Read the model definition and answer for the solid it produces. Units are mm, in the model's axes. A direction names the side the tool comes from. Coordinates: 2 decimals unless noted, no trailing zeros. Write each loop counter-clockwise with the first axis right and the second up, starting at its lowest first coordinate (ties: lowest second). Pieces come first, ordered by that corner, then holes. Notation, with made-up numbers: (40, -12.5) -> (79, -12.5) arc R13 cw to (79, -0.5) -> close; hole circle Ø10 at (-40, 56). An arc over 180 degrees is marked (long way). Answer in a Markdown table with one row per item. Add a question column.
Item 1: Which of the six approach directions +Z, -Z, +X, -X, +Y, -Y give full straight-line access (tool end or side, diameter ignored) to faces 1 (the face through (122, 13, -12.446)), 2 (the face through (122, 13, 10.414))?
Item 2: Section B-B on x = 267 is taken. Write down the section's boundary in (y, z), then the cut area to 3 significant figures.
Item 3: Given pin 1 Ø4 at (x, y) = (281.178, 12.7) entering from +Z, flat-ended and moving along its own axis, determine where the tip first touches the part or whether it passes through.
Item 4: For a pull along Y with two mould halves and no side action, classify faces 3 (the face through (122, 13, 12.954)), 4 (the face through (-75.18, 8.26, -11.16)), 5 (the face through (122, 2.54, 0)), 6 (the face through (122, 0, 0)) as +Y half, -Y half, draft (parallel to the pull), parting line (faces both ways), or undercut.
Item 5: Straight lines are drawn through the part: line 1 (Y direction, x = 123, z = -2.75); line 2 (Z direction, x = 214, y = 8.25); line 3 (X direction, y = 9, z = -11). For each, find the intervals that lie inside material, in ascending order. Write a range as from..to.
Item 6: Section A-A on z = -5.5 is taken. Write down the section's boundary in (x, y), then the cut area to 3 significant figures.
```python
from build123d import *

# Parameters (mm, degrees)
SKETCH1_W           = 431.8
SKETCH1_H           = 25.4
BOSS_EXTRUDE1_DEPTH = 25.4
SKETCH2_W           = 20.32
SKETCH2_H           = 20.32
CUT_EXTRUDE1_DEPTH  = 433.740344914
CUT_EXTRUDE2_REACH  = 344.058
SKETCH3_R           = 1.5875
CUT_EXTRUDE3_REACH  = 344.755
SKETCH4_R           = 3.175
SKETCH4_R_2         = 3.302


with BuildPart() as part:
    # Sketch1 → Boss-Extrude1 (new body)
    with BuildSketch(Plane(origin=(0, 0, 0), x_dir=(1, 0, 0), z_dir=(0, 1, 0))):
        with Locations((124.968, -0.254)):
            Rectangle(SKETCH1_W, SKETCH1_H)
    extrude(amount=BOSS_EXTRUDE1_DEPTH)

    # Sketch2 → Cut-Extrude1 (cut, through all)
    with BuildSketch(Plane.ZY.offset(90.932)):
        with Locations((0.254, 12.7)):
            Rectangle(SKETCH2_W, SKETCH2_H)
    extrude(amount=-CUT_EXTRUDE1_DEPTH, mode=Mode.SUBTRACT)

    # Cut-Extrude2: up to this face of the body (flat: up to its plane)
    cut_extrude2_end = Plane(part.part.faces().sort_by_distance((124.968, 12.7, -12.446))[0])
    # Sketch3 → Cut-Extrude2 (cut, up to the picked face)
    with BuildSketch(Plane(origin=(0, 12.446, 12.954), x_dir=(1, 0, 0), z_dir=(0, 0, -1)), mode=Mode.PRIVATE) as cut_extrude2_sk1:
        with Locations((-74.422, -0.254)):
            Circle(SKETCH3_R)
    cut_extrude2_tool1 = split(extrude(cut_extrude2_sk1.sketch, amount=CUT_EXTRUDE2_REACH, mode=Mode.PRIVATE), bisect_by=cut_extrude2_end, keep=Keep.BOTH, mode=Mode.PRIVATE)
    # Sketch3 → Cut-Extrude2 (cut, up to the picked face)
    with BuildSketch(Plane(origin=(0, 12.446, 12.954), x_dir=(1, 0, 0), z_dir=(0, 0, -1)), mode=Mode.PRIVATE) as cut_extrude2_sk2:
        with Locations((-49.022, -0.254)):
            Circle(SKETCH3_R)
    cut_extrude2_tool2 = split(extrude(cut_extrude2_sk2.sketch, amount=CUT_EXTRUDE2_REACH, mode=Mode.PRIVATE), bisect_by=cut_extrude2_end, keep=Keep.BOTH, mode=Mode.PRIVATE)
    # Sketch3 → Cut-Extrude2 (cut, up to the picked face)
    with BuildSketch(Plane(origin=(0, 12.446, 12.954), x_dir=(1, 0, 0), z_dir=(0, 0, -1)), mode=Mode.PRIVATE) as cut_extrude2_sk3:
        with Locations((-23.622, -0.254)):
            Circle(SKETCH3_R)
    cut_extrude2_tool3 = split(extrude(cut_extrude2_sk3.sketch, amount=CUT_EXTRUDE2_REACH, mode=Mode.PRIVATE), bisect_by=cut_extrude2_end, keep=Keep.BOTH, mode=Mode.PRIVATE)
    # Sketch3 → Cut-Extrude2 (cut, up to the picked face)
    with BuildSketch(Plane(origin=(0, 12.446, 12.954), x_dir=(1, 0, 0), z_dir=(0, 0, -1)), mode=Mode.PRIVATE) as cut_extrude2_sk4:
        with Locations((1.778, -0.254)):
            Circle(SKETCH3_R)
    cut_extrude2_tool4 = split(extrude(cut_extrude2_sk4.sketch, amount=CUT_EXTRUDE2_REACH, mode=Mode.PRIVATE), bisect_by=cut_extrude2_end, keep=Keep.BOTH, mode=Mode.PRIVATE)
    # Sketch3 → Cut-Extrude2 (cut, up to the picked face)
    with BuildSketch(Plane(origin=(0, 12.446, 12.954), x_dir=(1, 0, 0), z_dir=(0, 0, -1)), mode=Mode.PRIVATE) as cut_extrude2_sk5:
        with Locations((27.178, -0.254)):
            Circle(SKETCH3_R)
    cut_extrude2_tool5 = split(extrude(cut_extrude2_sk5.sketch, amount=CUT_EXTRUDE2_REACH, mode=Mode.PRIVATE), bisect_by=cut_extrude2_end, keep=Keep.BOTH, mode=Mode.PRIVATE)
    # Sketch3 → Cut-Extrude2 (cut, up to the picked face)
    with BuildSketch(Plane(origin=(0, 12.446, 12.954), x_dir=(1, 0, 0), z_dir=(0, 0, -1)), mode=Mode.PRIVATE) as cut_extrude2_sk6:
        with Locations((52.578, -0.254)):
            Circle(SKETCH3_R)
    cut_extrude2_tool6 = split(extrude(cut_extrude2_sk6.sketch, amount=CUT_EXTRUDE2_REACH, mode=Mode.PRIVATE), bisect_by=cut_extrude2_end, keep=Keep.BOTH, mode=Mode.PRIVATE)
    # Sketch3 → Cut-Extrude2 (cut, up to the picked face)
    with BuildSketch(Plane(origin=(0, 12.446, 12.954), x_dir=(1, 0, 0), z_dir=(0, 0, -1)), mode=Mode.PRIVATE) as cut_extrude2_sk7:
        with Locations((77.978, -0.254)):
            Circle(SKETCH3_R)
    cut_extrude2_tool7 = split(extrude(cut_extrude2_sk7.sketch, amount=CUT_EXTRUDE2_REACH, mode=Mode.PRIVATE), bisect_by=cut_extrude2_end, keep=Keep.BOTH, mode=Mode.PRIVATE)
    # Sketch3 → Cut-Extrude2 (cut, up to the picked face)
    with BuildSketch(Plane(origin=(0, 12.446, 12.954), x_dir=(1, 0, 0), z_dir=(0, 0, -1)), mode=Mode.PRIVATE) as cut_extrude2_sk8:
        with Locations((103.378, -0.254)):
            Circle(SKETCH3_R)
    cut_extrude2_tool8 = split(extrude(cut_extrude2_sk8.sketch, amount=CUT_EXTRUDE2_REACH, mode=Mode.PRIVATE), bisect_by=cut_extrude2_end, keep=Keep.BOTH, mode=Mode.PRIVATE)
    # Sketch3 → Cut-Extrude2 (cut, up to the picked face)
    with BuildSketch(Plane(origin=(0, 12.446, 12.954), x_dir=(1, 0, 0), z_dir=(0, 0, -1)), mode=Mode.PRIVATE) as cut_extrude2_sk9:
        with Locations((128.778, -0.254)):
            Circle(SKETCH3_R)
    cut_extrude2_tool9 = split(extrude(cut_extrude2_sk9.sketch, amount=CUT_EXTRUDE2_REACH, mode=Mode.PRIVATE), bisect_by=cut_extrude2_end, keep=Keep.BOTH, mode=Mode.PRIVATE)
    # Sketch3 → Cut-Extrude2 (cut, up to the picked face)
    with BuildSketch(Plane(origin=(0, 12.446, 12.954), x_dir=(1, 0, 0), z_dir=(0, 0, -1)), mode=Mode.PRIVATE) as cut_extrude2_sk10:
        with Locations((154.178, -0.254)):
            Circle(SKETCH3_R)
    cut_extrude2_tool10 = split(extrude(cut_extrude2_sk10.sketch, amount=CUT_EXTRUDE2_REACH, mode=Mode.PRIVATE), bisect_by=cut_extrude2_end, keep=Keep.BOTH, mode=Mode.PRIVATE)
    # Sketch3 → Cut-Extrude2 (cut, up to the picked face)
    with BuildSketch(Plane(origin=(0, 12.446, 12.954), x_dir=(1, 0, 0), z_dir=(0, 0, -1)), mode=Mode.PRIVATE) as cut_extrude2_sk11:
        with Locations((179.578, -0.254)):
            Circle(SKETCH3_R)
    cut_extrude2_tool11 = split(extrude(cut_extrude2_sk11.sketch, amount=CUT_EXTRUDE2_REACH, mode=Mode.PRIVATE), bisect_by=cut_extrude2_end, keep=Keep.BOTH, mode=Mode.PRIVATE)
    # Sketch3 → Cut-Extrude2 (cut, up to the picked face)
    with BuildSketch(Plane(origin=(0, 12.446, 12.954), x_dir=(1, 0, 0), z_dir=(0, 0, -1)), mode=Mode.PRIVATE) as cut_extrude2_sk12:
        with Locations((204.978, -0.254)):
            Circle(SKETCH3_R)
    cut_extrude2_tool12 = split(extrude(cut_extrude2_sk12.sketch, amount=CUT_EXTRUDE2_REACH, mode=Mode.PRIVATE), bisect_by=cut_extrude2_end, keep=Keep.BOTH, mode=Mode.PRIVATE)
    # Sketch3 → Cut-Extrude2 (cut, up to the picked face)
    with BuildSketch(Plane(origin=(0, 12.446, 12.954), x_dir=(1, 0, 0), z_dir=(0, 0, -1)), mode=Mode.PRIVATE) as cut_extrude2_sk13:
        with Locations((230.378, -0.254)):
            Circle(SKETCH3_R)
    cut_extrude2_tool13 = split(extrude(cut_extrude2_sk13.sketch, amount=CUT_EXTRUDE2_REACH, mode=Mode.PRIVATE), bisect_by=cut_extrude2_end, keep=Keep.BOTH, mode=Mode.PRIVATE)
    # Sketch3 → Cut-Extrude2 (cut, up to the picked face)
    with BuildSketch(Plane(origin=(0, 12.446, 12.954), x_dir=(1, 0, 0), z_dir=(0, 0, -1)), mode=Mode.PRIVATE) as cut_extrude2_sk14:
        with Locations((255.778, -0.254)):
            Circle(SKETCH3_R)
    cut_extrude2_tool14 = split(extrude(cut_extrude2_sk14.sketch, amount=CUT_EXTRUDE2_REACH, mode=Mode.PRIVATE), bisect_by=cut_extrude2_end, keep=Keep.BOTH, mode=Mode.PRIVATE)
    # Sketch3 → Cut-Extrude2 (cut, up to the picked face)
    with BuildSketch(Plane(origin=(0, 12.446, 12.954), x_dir=(1, 0, 0), z_dir=(0, 0, -1)), mode=Mode.PRIVATE) as cut_extrude2_sk15:
        with Locations((281.178, -0.254)):
            Circle(SKETCH3_R)
    cut_extrude2_tool15 = split(extrude(cut_extrude2_sk15.sketch, amount=CUT_EXTRUDE2_REACH, mode=Mode.PRIVATE), bisect_by=cut_extrude2_end, keep=Keep.BOTH, mode=Mode.PRIVATE)
    # Sketch3 → Cut-Extrude2 (cut, up to the picked face)
    with BuildSketch(Plane(origin=(0, 12.446, 12.954), x_dir=(1, 0, 0), z_dir=(0, 0, -1)), mode=Mode.PRIVATE) as cut_extrude2_sk16:
        with Locations((306.578, -0.254)):
            Circle(SKETCH3_R)
    cut_extrude2_tool16 = split(extrude(cut_extrude2_sk16.sketch, amount=CUT_EXTRUDE2_REACH, mode=Mode.PRIVATE), bisect_by=cut_extrude2_end, keep=Keep.BOTH, mode=Mode.PRIVATE)
    # Sketch3 → Cut-Extrude2 (cut, up to the picked face)
    with BuildSketch(Plane(origin=(0, 12.446, 12.954), x_dir=(1, 0, 0), z_dir=(0, 0, -1)), mode=Mode.PRIVATE) as cut_extrude2_sk17:
        with Locations((331.978, -0.254)):
            Circle(SKETCH3_R)
    cut_extrude2_tool17 = split(extrude(cut_extrude2_sk17.sketch, amount=CUT_EXTRUDE2_REACH, mode=Mode.PRIVATE), bisect_by=cut_extrude2_end, keep=Keep.BOTH, mode=Mode.PRIVATE)
    add(cut_extrude2_tool1.solids().sort_by(Axis((-74.422, 12.7, 12.954), (0, 0, -1)))[0], mode=Mode.SUBTRACT)
    add(cut_extrude2_tool2.solids().sort_by(Axis((-49.022, 12.7, 12.954), (0, 0, -1)))[0], mode=Mode.SUBTRACT)
    add(cut_extrude2_tool3.solids().sort_by(Axis((-23.622, 12.7, 12.954), (0, 0, -1)))[0], mode=Mode.SUBTRACT)
    add(cut_extrude2_tool4.solids().sort_by(Axis((1.778, 12.7, 12.954), (0, 0, -1)))[0], mode=Mode.SUBTRACT)
    add(cut_extrude2_tool5.solids().sort_by(Axis((27.178, 12.7, 12.954), (0, 0, -1)))[0], mode=Mode.SUBTRACT)
    add(cut_extrude2_tool6.solids().sort_by(Axis((52.578, 12.7, 12.954), (0, 0, -1)))[0], mode=Mode.SUBTRACT)
    add(cut_extrude2_tool7.solids().sort_by(Axis((77.978, 12.7, 12.954), (0, 0, -1)))[0], mode=Mode.SUBTRACT)
    add(cut_extrude2_tool8.solids().sort_by(Axis((103.378, 12.7, 12.954), (0, 0, -1)))[0], mode=Mode.SUBTRACT)
    add(cut_extrude2_tool9.solids().sort_by(Axis((128.778, 12.7, 12.954), (0, 0, -1)))[0], mode=Mode.SUBTRACT)
    add(cut_extrude2_tool10.solids().sort_by(Axis((154.178, 12.7, 12.954), (0, 0, -1)))[0], mode=Mode.SUBTRACT)
    add(cut_extrude2_tool11.solids().sort_by(Axis((179.578, 12.7, 12.954), (0, 0, -1)))[0], mode=Mode.SUBTRACT)
    add(cut_extrude2_tool12.solids().sort_by(Axis((204.978, 12.7, 12.954), (0, 0, -1)))[0], mode=Mode.SUBTRACT)
    add(cut_extrude2_tool13.solids().sort_by(Axis((230.378, 12.7, 12.954), (0, 0, -1)))[0], mode=Mode.SUBTRACT)
    add(cut_extrude2_tool14.solids().sort_by(Axis((255.778, 12.7, 12.954), (0, 0, -1)))[0], mode=Mode.SUBTRACT)
    add(cut_extrude2_tool15.solids().sort_by(Axis((281.178, 12.7, 12.954), (0, 0, -1)))[0], mode=Mode.SUBTRACT)
    add(cut_extrude2_tool16.solids().sort_by(Axis((306.578, 12.7, 12.954), (0, 0, -1)))[0], mode=Mode.SUBTRACT)
    add(cut_extrude2_tool17.solids().sort_by(Axis((331.978, 12.7, 12.954), (0, 0, -1)))[0], mode=Mode.SUBTRACT)

    # Cut-Extrude3: up to this face of the body (flat: up to its plane)
    cut_extrude3_end = Plane(part.part.faces().sort_by_distance((124.920663358, 12.7, -12.446))[0])
    # Sketch4 → Cut-Extrude3 (cut, up to the picked face)
    with BuildSketch(Plane.XY.offset(12.954), mode=Mode.PRIVATE) as cut_extrude3_sk1:
        with Locations((329.438, 12.763758165)):
            Circle(SKETCH4_R)
    cut_extrude3_tool1 = split(extrude(cut_extrude3_sk1.sketch, amount=-CUT_EXTRUDE3_REACH, mode=Mode.PRIVATE), bisect_by=cut_extrude3_end, keep=Keep.BOTH, mode=Mode.PRIVATE)
    # Sketch4 → Cut-Extrude3 (cut, up to the picked face)
    with BuildSketch(Plane.XY.offset(12.954), mode=Mode.PRIVATE) as cut_extrude3_sk2:
        with Locations((-78.232, 9.525)):
            Circle(SKETCH4_R_2)
    cut_extrude3_tool2 = split(extrude(cut_extrude3_sk2.sketch, amount=-CUT_EXTRUDE3_REACH, mode=Mode.PRIVATE), bisect_by=cut_extrude3_end, keep=Keep.BOTH, mode=Mode.PRIVATE)
    # Sketch4 → Cut-Extrude3 (cut, up to the picked face)
    with BuildSketch(Plane.XY.offset(12.954), mode=Mode.PRIVATE) as cut_extrude3_sk3:
        with Locations((-52.832, 9.525)):
            Circle(SKETCH4_R_2)
    cut_extrude3_tool3 = split(extrude(cut_extrude3_sk3.sketch, amount=-CUT_EXTRUDE3_REACH, mode=Mode.PRIVATE), bisect_by=cut_extrude3_end, keep=Keep.BOTH, mode=Mode.PRIVATE)
    add(cut_extrude3_tool1.solids().sort_by(Axis((329.438, 12.763758, 12.954), (0, 0, -1)))[0], mode=Mode.SUBTRACT)
    add(cut_extrude3_tool2.solids().sort_by(Axis((-78.232, 9.525, 12.954), (0, 0, -1)))[0], mode=Mode.SUBTRACT)
    add(cut_extrude3_tool3.solids().sort_by(Axis((-52.832, 9.525, 12.954), (0, 0, -1)))[0], mode=Mode.SUBTRACT)


solid = part.part
```
Results below:
| question | item | result |
|---|---|---|
| 1 | face 1 | -Z, +X, -X, +Y, -Y |
| 1 | face 2 | +X, -X |
| 2 | outline | (0, -12.45) -> (25.4, -12.45) -> (25.4, 12.95) -> (0, 12.95) -> close; hole (2.54, -9.91) -> (22.86, -9.91) -> (22.86, 10.41) -> (2.54, 10.41) -> close |
| 2 | area | 232 mm2 |
| 3 | pin 1 | stops at z = 12.95 |
| 4 | face 3 | draft |
| 4 | face 4 | undercut |
| 4 | face 5 | undercut |
| 4 | face 6 | -Y half |
| 5 | line 1 | y = 0..2.54, 22.86..25.4 |
| 5 | line 2 | z = -12.45..-9.91, 10.41..12.95 |
| 5 | line 3 | x = -90.93..-81.49, -74.97..-56.09, -49.57..340.87 |
| 6 | outline | (-90.93, 0) -> (340.87, 0) -> (340.87, 2.54) -> (-90.93, 2.54) -> close; (-90.93, 22.86) -> (340.87, 22.86) -> (340.87, 25.4) -> (-90.93, 25.4) -> close |
| 6 | area | 2,190 mm2 |
